```python
from build123d import *

# Parameters (mm, degrees)
SKETCH1_R           = 8.73125
BOSS_EXTRUDE1_DEPTH = 7.62
SKETCH2_R           = 2.7686
CUT_EXTRUDE1_DEPTH  = 3.81
CUT_EXTRUDE2_REACH  = 15.653
SKETCH3_R           = 1.7526


with BuildPart() as part:
    # Sketch1 → Boss-Extrude1 (new body)
    with BuildSketch(Plane(origin=(0, 0, 0), x_dir=(1, 0, 0), z_dir=(0, 1, 0))):
        Circle(SKETCH1_R)
        with BuildLine():
            Line((-2.032, 2.439590334), (2.032, 2.439590334))
            ThreePointArc((2.032, 2.439590334), (0, -3.175), (-2.032, 2.439590334))
        make_face(mode=Mode.SUBTRACT)
    extrude(amount=BOSS_EXTRUDE1_DEPTH)

    # Sketch2 → Cut-Extrude1 (cut)
    with BuildSketch(Plane(origin=(0, 0, -8.73125), x_dir=(-1, 0, 0), z_dir=(0, 0, -1))):
        with Locations((0, 4.064)):
            Circle(SKETCH2_R)
    extrude(amount=-CUT_EXTRUDE1_DEPTH, mode=Mode.SUBTRACT)

    # Sketch3 → Cut-Extrude2 (cut, up to next)
    with BuildSketch(Plane(origin=(0, 0, -4.92125), x_dir=(-1, 0, 0), z_dir=(0, 0, -1)), mode=Mode.PRIVATE) as cut_extrude2_sk1:
        with Locations((0, 4.064)):
            Circle(SKETCH3_R)
    cut_extrude2_tool1 = extrude(cut_extrude2_sk1.sketch, amount=-CUT_EXTRUDE2_REACH, mode=Mode.PRIVATE) & part.part
    add(cut_extrude2_tool1.solids().sort_by_distance((0, 4.064, -4.92125))[0], mode=Mode.SUBTRACT)


solid = part.part
```
Here's how the part is built. I have some questions about the finished solid (model axes, mm). A direction names the side the tool comes from. Coordinates: 2 decimals unless noted, no trailing zeros. Order: outer loops, then holes, each group sorted by start corner. A loop starts at its lowest first (then second) coordinate and runs counter-clockwise, first axis right, second up. Notation, with made-up numbers: (18.5, 87) - (70.5, 87) arc R6 ccw to (70.5, 94) - close; hole circle Ø8 at (-14, -0.75). An arc over 180 degrees is marked (long way). One line per question, with ' | ' between items. Start each with the question number.
1. I'm going to push flat-ended pins straight in: pin 1 Ø1 at (x, y) = (-3, 5) entering from +Z; pin 2 Ø1.7 at (x, y) = (0, 3.5) entering from -Z; pin 3 Ø7.5 at (x, z) = (0, 0) entering from -Y; pin 4 Ø1.5 at (x, y) = (2, 1.5) entering from -Z. Where does each tip first touch, or does it pass through?
2. If we section it at B-B (x = 0): Write out the boundary of the cut face in (y, z) (3 decimals).
3. Please list where these lines run through material, in increasing order: line 1 along Y through (x, z) = (0, -3.75); line 2 along Y through (x, z) = (0, -7.8); line 3 along X through (y, z) = (4.75, 0) (3 decimals). Write a range as [from, to].
4. If we section it at A-A (z = 0): Write out the boundary of the cut face in (x, y) (3 decimals).
5. If we section it at D-D (x = 7.75): Write out the boundary of the cut face in (y, z), and give its area (3 significant figures).
6. Which directions (+Z, -Z, +X, -X, +Y, -Y) give clear straight access to the entire face, cutting with the end or side of a thin tool? Please do faces 4 (the cylindrical face through (0.23, 5.8, -3.7)), 5 (the cylindrical face through (0.109, 3.757, 3.173)).
7. If we mould it in two halves opening along Z, with no side actions, what happens to faces 1 (the cylindrical face through (-1.893, 3.757, 8.524)), 2 (the cylindrical face through (-2.557, 3.004, -6.853)), 3 (the flat face through (0, 2, -2.44))? For each: released by +Z, released by -Z, zero draft, split by the parting line, or undercut.
Model answer:
1) pin 1: stops at z = 8.37 | pin 2: stops at z = 3.06 | pin 3: stops at y = 0 | pin 4: stops at z = -8.64
2) outline: (0, -8.731) - (1.295, -8.731) - (1.295, -4.921) - (2.311, -4.921) - (2.311, -2.44) - (0, -2.44) - close; (0, 3.175) - (7.62, 3.175) - (7.62, 8.731) - (0, 8.731) - close; (5.817, -4.921) - (6.833, -4.921) - (6.833, -8.731) - (7.62, -8.731) - (7.62, -2.44) - (5.817, -2.44) - close
3) line 1: y = [0, 2.31], [5.82, 7.62] | line 2: y = [0, 1.3], [6.83, 7.62] | line 3: x = [-8.731, -3.175], [3.175, 8.731]
4) outline: (-8.731, 0) - (-3.175, 0) - (-3.175, 7.62) - (-8.731, 7.62) - close; (3.175, 0) - (8.731, 0) - (8.731, 7.62) - (3.175, 7.62) - close
5) outline: (0, -4.02) - (7.62, -4.02) - (7.62, 4.02) - (0, 4.02) - close | area: 61.3 mm²
6) face 4: -Z | face 5: +Y, -Y
7) face 1: split by the parting line | face 2: zero draft | face 3: undercut
